from build123d import *

# Parameters (mm, degrees)
F1_DEPTH = 3.175
F2_W     = 3.175
F2_H     = 25.4
F3_DEPTH = 114.3
F4_W     = 3.175
F4_H     = 114.3
F4_W_2   = 19.05
F4_H_2   = 3.175
F5_DEPTH = 3.175
F6_D     = 6.35
F7_R     = 3.17499


# Not quite as in the source:
# - a fillet or chamfer is up to 0.001 mm smaller than in the source, because OpenCascade refuses the exact size


with BuildPart() as f1:
    # F0 (on Top) → F1 (new body)
    with BuildSketch(Plane.XY):
        with BuildLine():
            Line((34.925, 12.7), (-34.925, 12.7))
            ThreePointArc((-34.925, 12.7), (-37.1700640303, 11.7700640303), (-38.1, 9.525))
            Line((-38.1, 9.525), (-38.1, -9.525))
            ThreePointArc((-38.1, -9.525), (-37.1700640303, -11.7700640303), (-34.925, -12.7))
            Line((-34.925, -12.7), (34.925, -12.7))
            ThreePointArc((34.925, -12.7), (37.1700640303, -11.7700640303), (38.1, -9.525))
            Line((38.1, -9.525), (38.1, 9.525))
            ThreePointArc((38.1, 9.525), (37.1700640303, 11.7700640303), (34.925, 12.7))
        make_face()
        with BuildLine():
            Line((-34.925, -6.35), (-34.925, 6.35))
            ThreePointArc((-34.925, 6.35), (-31.75, 9.525), (-28.575, 6.35))
            Line((-28.575, 6.35), (-28.575, -6.35))
            ThreePointArc((-28.575, -6.35), (-31.75, -9.525), (-34.925, -6.35))
        make_face(mode=Mode.SUBTRACT)
        with BuildLine():
            Line((28.575, -6.35), (28.575, 6.35))
            ThreePointArc((28.575, 6.35), (31.75, 9.525), (34.925, 6.35))
            Line((34.925, 6.35), (34.925, -6.35))
            ThreePointArc((34.925, -6.35), (31.75, -9.525), (28.575, -6.35))
        make_face(mode=Mode.SUBTRACT)
    extrude(amount=F1_DEPTH)

    # F2 (on face) → F3 (join)
    with BuildSketch(Plane.XY.offset(3.175)):
        with Locations((11.1125, 0)):
            Rectangle(F2_W, F2_H)
        with Locations((-11.1125, 0)):
            Rectangle(F2_W, F2_H)
    extrude(amount=F3_DEPTH)

    # F4 (on face) → F5 (join)
    with BuildSketch(Plane(origin=(0, 12.7, 0), x_dir=(-1, 0, 0), z_dir=(0, 1, 0))):
        with Locations((-11.1125, 60.325)):
            Rectangle(F4_W, F4_H)
        with Locations((0, 60.325)):
            Rectangle(F4_W_2, F4_H)
        with Locations((11.1125, 60.325)):
            Rectangle(F4_W, F4_H)
        with Locations((0, 1.5875)):
            Rectangle(F4_W_2, F4_H_2)
        with Locations((-11.1125, 1.5875)):
            Rectangle(F4_W, F4_H_2)
        with Locations((11.1125, 1.5875)):
            Rectangle(F4_W, F4_H_2)
    extrude(amount=F5_DEPTH)

    # F6 (through all)
    with Locations(Plane(origin=(0, 12.7, 0), x_dir=(-1, 0, 0), z_dir=(0, -1, 0))):
        with Locations((0, -28.575), (0, -60.325), (0, -92.075)):
            Hole(F6_D / 2)

    # F7 (radius 3.175 in the source; OpenCascade refuses exactly that, so slightly less here)
    f7_edges = [f1.edges().sort_by_distance(p)[0] for p in [
        (0, 15.875, 0),
        (12.7, 15.875, 58.7375),
        (-12.7, 15.875, 58.7375),
    ]]
    fillet(f7_edges, radius=F7_R)


solid = f1.part
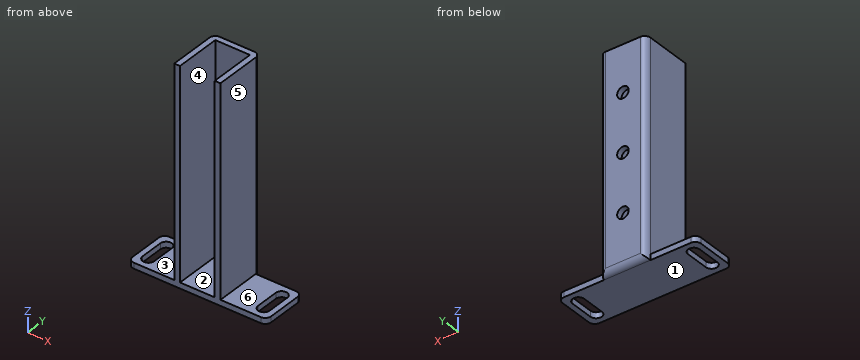
Model file for the job. Use its own axes, mm. Face numbers are marked on the shaded views. A direction names the side the tool comes from. Give positions to 0.01 mm unless a question says otherwise; leave off trailing zeros. Write each loop counter-clockwise with the first axis right and the second up, starting at its lowest first coordinate (ties: lowest second). Pieces come first, ordered by that corner, then holes. Notation, with made-up numbers: (89.5, -19) -> (145.5, -19) arc R15 ccw to (145.5, 7) -> close; hole circle Ø2 at (-35, 58). An arc over 180 degrees is marked (long way). Write item = value, one per line.
(1) Slice it at B-B, the plane x = 31.75. Give the cut face in (y, z) (3 decimals).
Determined:
outline = (-12.7, 0) -> (-9.525, 0) -> (-9.525, 3.175) -> (-12.7, 3.175) -> close; (9.525, 0) -> (12.7, 0) -> (12.7, 3.175) -> (9.525, 3.175) -> close
(2) Slice it at D-D, the plane z = 101.5. Give the cut face in (x, y) (3 decimals), then the cut area to 3 significant figures.
Determined:
outline = (-12.7, -12.7) -> (-9.525, -12.7) -> (-9.525, 12.7) -> (9.525, 12.7) -> (9.525, -12.7) -> (12.7, -12.7) -> (12.7, 12.7) arc R3.175 ccw to (9.525, 15.875) -> (-9.525, 15.875) arc R3.175 ccw to (-12.7, 12.7) -> close
area = 238 mm2
(3) Slice it at C-C, the plane y = 4.75. Give the cut face in (x, z) (3 decimals).
Determined:
outline = (-38.1, 0) -> (-34.925, 0) -> (-34.925, 3.175) -> (-38.1, 3.175) -> close; (-28.575, 0) -> (28.575, 0) -> (28.575, 3.175) -> (12.7, 3.175) -> (12.7, 117.475) -> (9.525, 117.475) -> (9.525, 3.175) -> (-9.525, 3.175) -> (-9.525, 117.475) -> (-12.7, 117.475) -> (-12.7, 3.175) -> (-28.575, 3.175) -> close; (34.925, 0) -> (38.1, 0) -> (38.1, 3.175) -> (34.925, 3.175) -> close
(4) Flat gauge pins, fed straight in: P1, Ø8.5, axis at x = 0, z = 60.325, coming from the -Y side; P2, Ø1.5, axis at x = -2.5, y = -5.5, coming from the +Z side (3 decimals); P3, Ø7.5, axis at y = -3, z = 50, coming from the -X side. Where does each tip first touch, or does it go through?
Determined:
P1 = 12.7
P2 = 3.175
P3 = -12.7
(5) Probe line 1 along X through (y, z) = (1, 38) (3 decimals); line 2 along Z through (x, y) = (0, 14.4) (3 decimals); line 3 along Z through (x, y) = (0, 13.55) (3 decimals). List the from-to ranges inside material, lowest first.
Determined:
line_1 = -12.7 to -9.525, 9.525 to 12.7
line_2 = 0.493 to 25.4, 31.75 to 57.15, 63.5 to 88.9, 95.25 to 117.475
line_3 = 0.116 to 25.4, 31.75 to 57.15, 63.5 to 88.9, 95.25 to 117.475
(6) Tool access for the marked faces 1, 2 and 3: list every direction of +Z, -Z, +X, -X, +Y, -Y with a clear straight run to the whole face (end or side of a thin tool).
Determined:
face_1 = -Z, +X, -X, +Y, -Y
face_2 = +Z, -Y
face_3 = +Z, -X, +Y, -Y
(7) Mould opens along X. For the marked faces 4, 5 and 6 say: released by +X, released by -X, zero draft, split by the parting line, or undercut.
Determined:
face_4 = undercut
face_5 = released by +X
face_6 = zero draft
(8) Slice it at A-A, the plane x = 0. Give the cut face in (y, z) (3 decimals).
Determined:
outline = (-12.7, 0) -> (12.7, 0) arc R3.175 ccw to (15.875, 3.175) -> (15.875, 25.4) -> (12.7, 25.4) -> (12.7, 3.175) -> (-12.7, 3.175) -> close; (12.7, 31.75) -> (15.875, 31.75) -> (15.875, 57.15) -> (12.7, 57.15) -> close; (12.7, 63.5) -> (15.875, 63.5) -> (15.875, 88.9) -> (12.7, 88.9) -> close; (12.7, 95.25) -> (15.875, 95.25) -> (15.875, 117.475) -> (12.7, 117.475) -> close
